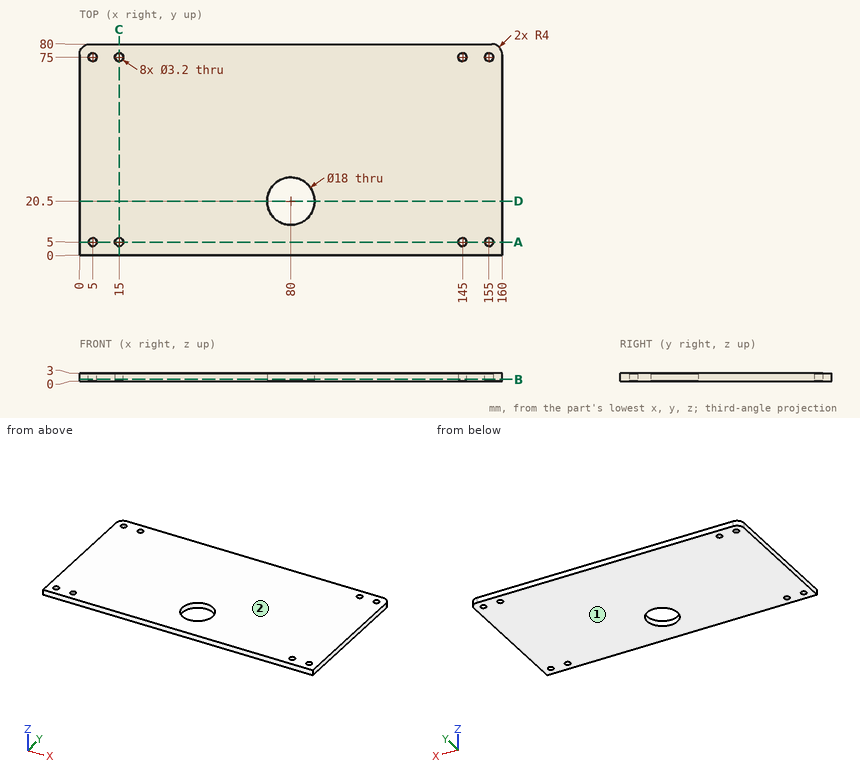
Design review of the part shown in the three views and the two pictorial views. Dimensions are in mm from the part's minimum x, y and z. Give positions to 0.01 mm unless a question says otherwise; leave off trailing zeros. Write each loop counter-clockwise with the first axis right and the second up, starting at its lowest first coordinate (ties: lowest second). Pieces come first, ordered by that corner, then holes. Notation, with made-up numbers: M 84.25,13.5 L 135.25,13.5 A19 cw 135.25,47.5 Z; hole C 89,34 d4. An arc over 180 degrees is marked long. One line per question, with ' | ' between items. Start each with the question number.
Item 1: We need section A-A on y = 5. Write out the cut boundary in (x, z).
Item 2: We need section C-C on x = 15. Write out the cut boundary in (y, z), plus the area to 3 significant figures.
Item 3: Wall thickness on line 1 (Y direction, x = 5, z = 1); line 2 (X direction, y = 5, z = 1.35); line 3 (X direction, y = 21, z = 1.65): over which ranges is each line inside the solid? List them lowest first. Write a range as from..to.
Item 4: Draft analysis for pull direction Z (two halves, no side actions). For the marked faces 1 and 2, state which applies: released by +Z, released by -Z, zero draft, split by the parting line, or undercut.
Item 5: For pin 1 (16 mm diameter, centred on x = 80, y = 20.5, fed in from -Z); pin 2 (4 mm diameter, centred on x = 145, y = 5, fed in from -Z), all flat-tipped, find the tip position at first contact; note any pin that passes through.
Item 6: We need section B-B on z = 0.7. Give the number of separate pieces and of enclosed holes in the cut face, plus the area to 3 significant figures.
Item 7: We need section D-D on y = 20.5. Write out the cut boundary in (x, z).
Results found:
1) outline: M 0,0 L 3.4,0 L 3.4,3 L 0,3 Z; M 6.6,0 L 13.4,0 L 13.4,3 L 6.6,3 Z; M 16.6,0 L 143.4,0 L 143.4,3 L 16.6,3 Z; M 146.6,0 L 153.4,0 L 153.4,3 L 146.6,3 Z; M 156.6,0 L 160,0 L 160,3 L 156.6,3 Z
2) outline: M 0,0 L 3.4,0 L 3.4,3 L 0,3 Z; M 6.6,0 L 73.4,0 L 73.4,3 L 6.6,3 Z; M 76.6,0 L 80,0 L 80,3 L 76.6,3 Z | area: 221 mm2
3) line 1: y = 0..3.4, 6.6..73.4, 76.6..80 | line 2: x = 0..3.4, 6.6..13.4, 16.6..143.4, 146.6..153.4, 156.6..160 | line 3: x = 0..71.01, 88.99..160
4) face 1: released by -Z | face 2: released by +Z
5) pin 1: passes through | pin 2: stops at z = 0
6) separate pieces: 1 | enclosed holes: 9 | area: 12,500 mm2
7) outline: M 0,0 L 71,0 L 71,3 L 0,3 Z; M 89,0 L 160,0 L 160,3 L 89,3 Z
